Verification items for this drawing (mm, ordinates from the low corner). A direction names the side the tool comes from. Coordinates: 2 decimals unless noted, no trailing zeros. Loops run counter-clockwise (first coordinate to the right, second up) from the corner with the lowest first, then second, coordinate; pieces in that order, holes last. Notation, with made-up numbers: M 71.25,80.25 L 118.25,80.25 A24 ccw 118.25,113.25 Z; hole C 82,-32 d3. An arc over 180 degrees is marked long. Return JSON: item names as keys, results as strings.
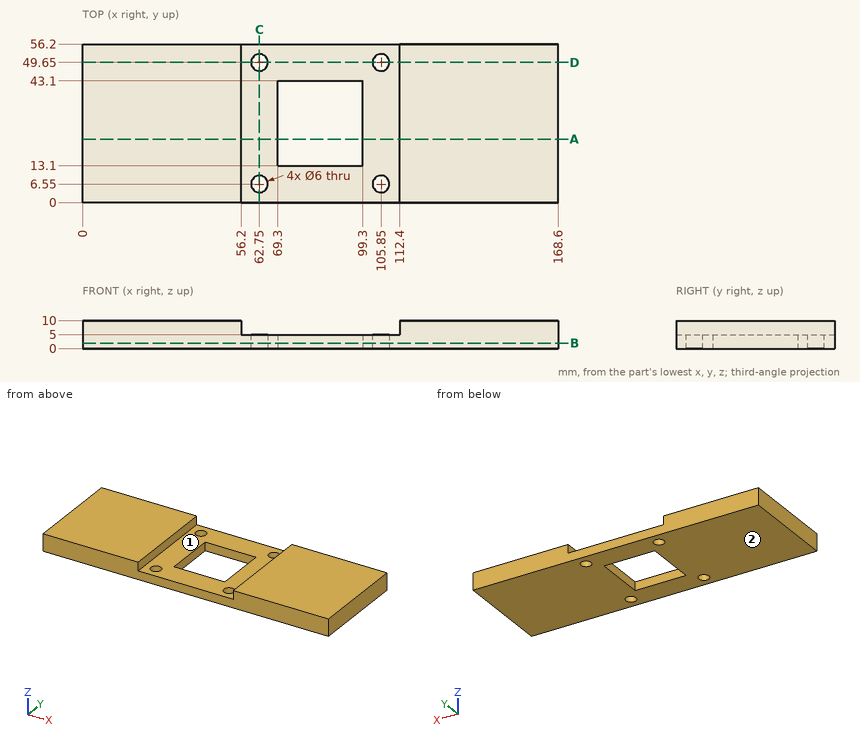
1) Section check D-D on y = 49.65. Record the cut outline in (x, z).
Answers:
{"outline": "M 0,0 L 59.75,0 L 59.75,5 L 56.2,5 L 56.2,10 L 0,10 Z; M 65.75,0 L 102.85,0 L 102.85,5 L 65.75,5 Z; M 108.85,0 L 168.6,0 L 168.6,10 L 112.4,10 L 112.4,5 L 108.85,5 Z"}
2) Scan lines: line 1 along Y through (x, z) = (105.85, 2); line 2 along X through (y, z) = (20, 0.5); line 3 along X through (y, z) = (16, 7.5). Record each from-to range of solid material in increasing order. Write a range as [from, to].
Answers:
{"line 1": "[0, 3.55], [9.55, 46.65], [52.65, 56.2]", "line 2": "[0, 69.3], [99.3, 168.6]", "line 3": "[0, 56.2], [112.4, 168.6]"}
3) Section check C-C on x = 62.75. Record the cut outline in (y, z), then the cut area to 3 significant figures.
Answers:
{"outline": "M 0,0 L 3.55,0 L 3.55,5 L 0,5 Z; M 9.55,0 L 46.65,0 L 46.65,5 L 9.55,5 Z; M 52.65,0 L 56.2,0 L 56.2,5 L 52.65,5 Z", "area": "221 mm²"}
4) Section check B-B on z = 2. Record the cut outline in (x, y).
Answers:
{"outline": "M 0,0 L 168.6,0 L 168.6,56.2 L 0,56.2 Z; hole C 62.75,6.55 d6; hole C 62.75,49.65 d6; hole M 69.3,13.1 L 99.3,13.1 L 99.3,43.1 L 69.3,43.1 Z; hole C 105.85,6.55 d6; hole C 105.85,49.65 d6"}
5) Go/stop test with flat-tipped pins: pin 1 Ø1.5 at (y, z) = (24, 1.5) entering from -X; pin 2 Ø9.5 at (x, y) = (105.85, 6.55) entering from +Z. Record where each tip stops, or that it passes through.
Answers:
{"pin 1": "x = 0", "pin 2": "z = 5"}
6) Section check A-A on y = 22.5. Record the cut outline in (x, z).
Answers:
{"outline": "M 0,0 L 69.3,0 L 69.3,5 L 56.2,5 L 56.2,10 L 0,10 Z; M 99.3,0 L 168.6,0 L 168.6,10 L 112.4,10 L 112.4,5 L 99.3,5 Z"}
7) Set-up check for the marked faces 1 and 2: record each of +Z, -Z, +X, -X, +Y, -Y from which the full face is reachable in a straight line by a thin tool's end or side.
Answers:
{"face 1": "+Z, +Y, -Y", "face 2": "-Z, +X, -X, +Y, -Y"}
